Design review of the part built by this model. Coordinates are the model's own, in mm. A direction names the side the tool comes from. Round coordinates to 2 decimals unless told otherwise and drop trailing zeros. Write each loop counter-clockwise with the first axis right and the second up, starting at its lowest first coordinate (ties: lowest second). Pieces come first, ordered by that corner, then holes. Notation, with made-up numbers: M -32,66 L 7,66 A15 cw 7,94 Z; hole C -28.75,13 d3. An arc over 180 degrees is marked long. One line per question, with ' | ' between items. Start each with the question number.
Item 1: Draft analysis for pull direction Z (two halves, no side actions). For faces 3 (the face through (-42.062, 765, 369)), 4 (the face through (-40.45, 749.56, 502.65)), 5 (the face through (-40.5, 820.58, 343.94)), 6 (the face through (-40.45, 779.25, 487.35)), state which applies: released by +Z, released by -Z, zero draft, split by the parting line, or undercut.
Item 2: Machinability: for faces 1 (the face through (-40.5, 788.8, 394.37)), 2 (the face through (-38.887, 765, 369)), which of the approach directions +Z, -Z, +X, -X, +Y, -Y give a long, thin tool a straight path to every point of the face, cutting with its end or side? Answer none if there is none.
Item 3: Add section C-C, the plane z = 255.5. State the section outline as (x, y) points, and give its area (3 significant figures).
Item 4: Add section A-A, the plane z = 502.5. State the section outline as (x, y) points.
Item 5: Insertion check: pin 1 Ø7.5 at (y, z) = (744.8, 526.09) entering from -X; pin 2 Ø1 at (x, z) = (-41, 249) entering from -Y; pin 3 Ø1.5 at (x, z) = (-41.5, 391) entering from -Y; pin 4 Ø1.6 at (x, y) = (-40, 807) entering from -Z. Each pin has a flat end and moves straight along its axis. Give the tip position at first contact, or say it passes through.
Item 6: For L1, parallel to Y at x = -40.8, z = 411; L2, parallel to Y at x = -41.8, z = 226.5; L3, parallel to Z at x = -40.4, y = 787.5, list the stretches that pass through material, from the lowest coordinate up.
Item 7: Add section D-D, the plane x = -41.15. Give the number of separate pieces and of enclosed holes in the cut face, and give its area (3 significant figures).
Item 8: Add section B-B, the plane y = 802. State the section outline as (x, z) points, and give its area (3 significant figures).
```python
from build123d import *

# Parameters (mm, degrees)
SKETCH1_R           = 3.175
SKETCH1_R_2         = 2.38125
SKETCH1_R_3         = 12.7
SKETCH1_R_4         = 3.175000001
SKETCH1_R_5         = 2.0193
SKETCH1_R_6         = 14.287500001
BOSS_EXTRUDE1_DEPTH = 3.175
FILLET1_R           = 12.7
FILLET2_R           = 6.35


with BuildPart() as part:
    # Sketch1 → Boss-Extrude1 (new body)
    with BuildSketch(Plane.ZY.offset(38.887083386)):
        with BuildLine():
            Line((342.127458156, 784.981140976), (200.726675, 784.981140976))
            Line((200.726675, 784.981140976), (200.726675, 740.531140976))
            Line((200.726675, 740.531140976), (342.992469809, 740.531140976))
            ThreePointArc((342.992469809, 740.531140976), (366.437970398, 754.238128734), (389.883470986, 740.531140976))
            Line((389.883470986, 740.531140976), (475.74833758, 740.531140976))
            ThreePointArc((475.74833758, 740.531140976), (480.3857219, 739.654197546), (484.382677289, 737.144474309))
            ThreePointArc((484.382677289, 737.144474309), (543.052111491, 762.756140976), (484.382677289, 788.367807643))
            ThreePointArc((484.382677289, 788.367807643), (480.3857219, 785.858084405), (475.74833758, 784.981140976))
            Line((475.74833758, 784.981140976), (390.74848264, 784.981140976))
            Line((390.74848264, 784.981140976), (390.74848264, 822.48966546))
            Line((390.74848264, 822.48966546), (342.127458156, 822.48966546))
            Line((342.127458156, 822.48966546), (342.127458156, 784.981140976))
        make_face()
        with Locations(Location((226.126675, 745.293640976, 0), (0, 0, 270))):
            Circle(SKETCH1_R, mode=Mode.SUBTRACT)
        with Locations(Location((308.3258375, 745.293640976, 0), (0, 0, 270))):
            Circle(SKETCH1_R, mode=Mode.SUBTRACT)
        with Locations(Location((226.126675, 780.218640976, 0), (0, 0, 270))):
            Circle(SKETCH1_R, mode=Mode.SUBTRACT)
        with Locations(Location((308.3258375, 780.218640976, 0), (0, 0, 270))):
            Circle(SKETCH1_R, mode=Mode.SUBTRACT)
        with Locations(Location((205.489175, 780.218640976, 0), (0, 0, 270))):
            Circle(SKETCH1_R, mode=Mode.SUBTRACT)
        with Locations(Location((205.489175, 745.293640976, 0), (0, 0, 270))):
            Circle(SKETCH1_R, mode=Mode.SUBTRACT)
        with Locations(Location((384.39848264, 780.218640976, 0), (0, 0, 270))):
            Circle(SKETCH1_R_2, mode=Mode.SUBTRACT)
        with Locations(Location((348.477458156, 780.218640976, 0), (0, 0, 270))):
            Circle(SKETCH1_R_2, mode=Mode.SUBTRACT)
        with Locations(Location((384.39848264, 816.13966546, 0), (0, 0, 270))):
            Circle(SKETCH1_R_2, mode=Mode.SUBTRACT)
        with Locations(Location((366.437970398, 798.179153218, 0), (0, 0, 270))):
            Circle(SKETCH1_R_3, mode=Mode.SUBTRACT)
        with Locations(Location((348.477458156, 816.13966546, 0), (0, 0, 270))):
            Circle(SKETCH1_R_2, mode=Mode.SUBTRACT)
        with Locations(Location((411.1625, 780.218640976, 0), (0, 0, 270))):
            Circle(SKETCH1_R, mode=Mode.SUBTRACT)
        with Locations(Location((411.1625, 745.293640976, 0), (0, 0, 270))):
            Circle(SKETCH1_R, mode=Mode.SUBTRACT)
        with Locations(Location((526.087623733, 780.716653218, 0), (0, 0, 270))):
            Circle(SKETCH1_R_4, mode=Mode.SUBTRACT)
        with Locations(Location((490.166599249, 744.795628734, 0), (0, 0, 270))):
            Circle(SKETCH1_R_4, mode=Mode.SUBTRACT)
        with Locations(Location((468.527325029, 746.353372356, 0), (0, 0, 270))):
            Circle(SKETCH1_R_5, mode=Mode.SUBTRACT)
        with Locations(Location((477.327277576, 749.998432049, 0), (0, 0, 270))):
            Circle(SKETCH1_R_5, mode=Mode.SUBTRACT)
        with Locations(Location((526.087623733, 744.795628734, 0), (0, 0, 270))):
            Circle(SKETCH1_R_4, mode=Mode.SUBTRACT)
        with Locations(Location((422.275, 762.756140976, 0), (0, 0, 270))):
            Circle(SKETCH1_R, mode=Mode.SUBTRACT)
        with Locations(Location((508.127111491, 762.756140976, 0), (0, 0, 270))):
            Circle(SKETCH1_R_6, mode=Mode.SUBTRACT)
        with Locations(Location((490.166599249, 780.716653218, 0), (0, 0, 270))):
            Circle(SKETCH1_R_4, mode=Mode.SUBTRACT)
    extrude(amount=BOSS_EXTRUDE1_DEPTH)

    # Fillet1
    fillet1_edges = [part.edges().sort_by_distance(p)[0] for p in [
        (-40.474583386, 784.981140976, 342.127458156),
        (-40.474583386, 784.981140976, 390.74848264),
        (-40.474583386, 740.531140976, 389.883470986),
        (-40.474583386, 740.531140976, 342.992469809),
    ]]
    fillet(fillet1_edges, radius=FILLET1_R)

    # Fillet2
    fillet2_edges = [part.edges().sort_by_distance(p)[0] for p in [
        (-40.474583386, 822.48966546, 342.127458156),
        (-40.474583386, 822.48966546, 390.74848264),
    ]]
    fillet(fillet2_edges, radius=FILLET2_R)


solid = part.part
```
Computed values:
1) face 3: zero draft | face 4: undercut | face 5: released by -Z | face 6: undercut
2) face 1: +X, -X, +Y | face 2: +Z, -Z, +X, +Y, -Y
3) outline: M -42.06,740.53 L -38.89,740.53 L -38.89,784.98 L -42.06,784.98 Z | area: 141 mm^2
4) outline: M -42.06,728.29 L -38.89,728.29 L -38.89,749.62 L -42.06,749.62 Z; M -42.06,775.89 L -38.89,775.89 L -38.89,797.22 L -42.06,797.22 Z
5) pin 1: stops at x = -42.06 | pin 2: stops at y = 740.53 | pin 3: stops at y = 741.41 | pin 4: stops at z = 342.13
6) L1: y = 740.53 to 742.12, 748.46 to 777.05, 783.39 to 784.98 | L2: y = 740.53 to 742.14, 748.45 to 777.07, 783.37 to 784.98 | L3: z = 337.02 to 359.56, 373.31 to 395.86, 483.34 to 532.77
7) separate pieces: 1 | enclosed holes: 21 | area: 15,800 mm^2
8) outline: M -42.06,342.13 L -38.89,342.13 L -38.89,354.33 L -42.06,354.33 Z; M -42.06,378.55 L -38.89,378.55 L -38.89,390.75 L -42.06,390.75 Z | area: 77.5 mm^2
